Geometry check sheet. Reference: the model listing, model coordinates, mm. A direction names the side the tool comes from. Give positions to 0.01 mm unless a question says otherwise; leave off trailing zeros. Loops run counter-clockwise (first coordinate to the right, second up) from the corner with the lowest first, then second, coordinate; pieces in that order, holes last.
1. Cross-section at B-B, the plane x = 11.2. Record the cut outline in (y, z).
2. Material ranges on L1, parallel to Y at x = 8.5, z = 2; L2, parallel to Z at x = -11.2, y = 2.35 (3 decimals); L3, parallel to X at y = 2.35, z = 0, recorded low to high.
3. Go/stop test with flat-tipped pins: pin 1 Ø2.5 at (x, z) = (11.2, 0) entering from +Y; pin 2 Ø3 at (y, z) = (-9.5, -14) entering from -X; pin 3 Ø1 at (x, y) = (7.5, 2) entering from -Z; pin 4 Ø1.5 at (x, y) = (18, 2.5) entering from -Z. Record where each tip stops, or that it passes through.
4. Cross-section at C-C, the plane y = 1.5. State how many separate pieces and enclosed holes the cut face has, plus the area to 3 significant figures.
5. Tool access check on faces 5 (the flat face through (1, -9, -4)), 6 (the flat face through (15, 5, -2)). Record the directions out of +Z, -Z, +X, -X, +Y, -Y that give a thin tool (end or side, any length) a straight path to the whole face; none if there is none.
6. Cross-section at A-A, the plane x = -7.5. Record the cut outline in (y, z), plus the area to 3 significant figures.
7. Release check for a two-part mould opening along Z. For faces 1 (the cylindrical face through (9.614, 2.516, 0.208)), 2 (the cylindrical face through (-13.859, -8.516, 2.797)), 3 (the cylindrical face through (-13.859, 2.584, -2.797)), 4 (the cylindrical face through (-9.614, 2.516, -0.208)) record: +Z half, -Z half, draft (parallel to the pull), parting line (faces both ways), or undercut.
from build123d import *
from build123d.topology import SkipClean

# Parameters (mm, degrees)
SKETCH_1_W               = 30
SKETCH_1_H               = 8
SKETCH_1_R               = 1.6
EXTRUDE_1_DEPTH          = 5
EXTRUDE_2_DEPTH          = 5
EXTRUDE_START            = 11
SKETCH_3_R               = 1.6
EXTRUDE_3_DEPTH          = 11
CUT_EXTRUDE_1_DEPTH      = 0.1
CUT_EXTRUDE_1_DEPTH_BACK = 6.1
FILLET_1_R               = 4
FILLET_2_R               = 4
CUT_EXTRUDE_2_DEPTH      = 16
FILLET_3_R               = 3
FILLET_4_R               = 5


# Some blends are built 0.0001 mm under size
with BuildPart() as part:
    # 草图1 → 凸台-拉伸1 (new body)
    with BuildSketch(Plane(origin=(0, 0, 0), x_dir=(1, 0, 0), z_dir=(0, 1, 0))):
        Rectangle(SKETCH_1_W, SKETCH_1_H)
        with Locations(Location((-11.2, 0, 0), (0, 0, 270))):
            Circle(SKETCH_1_R, mode=Mode.SUBTRACT)
        with Locations(Location((11.2, 0, 0), (0, 0, 90))):
            Circle(SKETCH_1_R, mode=Mode.SUBTRACT)
    extrude(amount=EXTRUDE_1_DEPTH)

    # 草图2 → 凸台-拉伸2 (add)
    with BuildSketch(Plane(origin=(0, 5, 0), x_dir=(1, 0, 0), z_dir=(0, 1, 0))):
        Polygon((15, 4), (41.779934935, 17.521652446), (44.998681359, 11.146853201), (15, -4), align=None)
    extrude(amount=-EXTRUDE_2_DEPTH)

    # 草图3 → 凸台-拉伸3 (add)
    with SkipClean():  # the faces are left unmerged after this step: merging them gives an invalid solid
        with BuildSketch(Plane.XZ.offset(EXTRUDE_START)):
            Polygon((-15, -4), (15, -4), (41.779934935, -17.521652446), (44.998681359, -11.146853201), (15, 4), (-15, 4), align=None)
            with Locations(Location((-11.2, 0, 0), (0, 0, 270))):
                Circle(SKETCH_3_R, mode=Mode.SUBTRACT)
            with Locations(Location((11.2, 0, 0), (0, 0, 270))):
                Circle(SKETCH_3_R, mode=Mode.SUBTRACT)
        extrude(amount=-EXTRUDE_3_DEPTH)

    # 草图4 → 切除-拉伸1 (cut, two sides: drawn at the far end of the back side and taken through both)
    with BuildSketch(Plane(origin=(0, 0, 0), x_dir=(1, 0, 0), z_dir=(0, 1, 0)).offset(-CUT_EXTRUDE_1_DEPTH_BACK)):
        Polygon((17.677993493, 5.352165245), (20.899244527, -1.027594436), (19.919281017, -1.51616991), (15, -4), (-15, -4), (-15, 4), (15, 4), align=None)
    extrude(amount=CUT_EXTRUDE_1_DEPTH + CUT_EXTRUDE_1_DEPTH_BACK, mode=Mode.SUBTRACT)

    # 圆角1
    fillet_1_edges = [part.edges().sort_by_distance(p)[0] for p in [
        (-15, -8.55, -4),
        (-15, 2.55, -4),
        (-15, -8.55, 4),
        (-15, 2.55, 4),
    ]]
    fillet(fillet_1_edges, radius=FILLET_1_R - 0.0001)  # a hair under: the kernel refuses the full size

    # 圆角2
    # the kernel refuses this fillet: 4 mm, written as the material it takes off along each edge
    with BuildSketch(Plane(origin=(41.779934935, 15, -17.521652446), x_dir=(-0.8926644978329522, 0, 0.45072174820907335), z_dir=(0, -1, 0)), Plane(origin=(44.998681359, -21, -11.146853201), x_dir=(-0.8926644978329524, 0, 0.450721748209073), z_dir=(0, 1, 0))) as fillet_2_piece_1:
        with BuildLine():
            CenterArc((FILLET_2_R, -FILLET_2_R), FILLET_2_R, 90, 90)
            Line((0, -FILLET_2_R), (0, 0))
            Line((0, 0), (FILLET_2_R, 0))
        make_face()
    extrude(amount=36, mode=Mode.SUBTRACT)

    # 草图5 → 切除-拉伸2 (cut)
    with BuildSketch(Plane(origin=(0, 5, 0), x_dir=(1, 0, 0), z_dir=(0, 1, 0))):
        with BuildLine():
            Line((20.896739918, -1.022634001), (41.428023368, 9.343966208))
            add(Edge.make_bspline(
                [(20.896739918, -1.022634001), (25.980191779, 4.72849772), (33.095529518, 10.551057562), (41.428023368, 9.343966208)],
                knots=[0, 0, 0, 0, 1, 1, 1, 1], degree=3))
        make_face()
    extrude(amount=-CUT_EXTRUDE_2_DEPTH, mode=Mode.SUBTRACT)

    # 圆角3
    fillet_3_edges = [part.edges().sort_by_distance(p)[0] for p in [
        (41.428023368, -3, -9.343966208),
    ]]
    fillet(fillet_3_edges, radius=FILLET_3_R)

    # 圆角4
    fillet_4_edges = [part.edges().sort_by_distance(p)[0] for p in [
        (15, -8.55, 4),
        (15, -8.55, -4),
        (15, 2.55, 4),
        (15, 2.55, -4),
    ]]
    fillet(fillet_4_edges, radius=FILLET_4_R)


solid = part.part
Result:
1. outline: (-11, -4) - (-6.1, -4) - (-6.1, -1.6) - (-11, -1.6) - close; (-11, 1.6) - (-6.1, 1.6) - (-6.1, 4) - (-11, 4) - close; (0.1, -4) - (5, -4) - (5, -1.6) - (0.1, -1.6) - close; (0.1, 1.6) - (5, 1.6) - (5, 4) - (0.1, 4) - close
2. L1: y = -11 to -6.1, 0.1 to 5
2. L2: z = -3.995 to -1.6, 1.6 to 3.995
2. L3: x = -15 to -12.8, -9.6 to 9.6, 12.8 to 21.82
3. pin 1: passes through
3. pin 2: stops at x = 31.83
3. pin 3: stops at z = -4
3. pin 4: stops at z = -5.89
4. separate pieces: 1
4. enclosed holes: 2
4. area: 392 mm2
5. face 5: -Z, -X, +Y, -Y
5. face 6: +Z, -Z, +X, -X, +Y
6. outline: (-11, -4) - (-6.1, -4) - (-6.1, 4) - (-11, 4) - close; (0.1, -4) - (5, -4) - (5, 4) - (0.1, 4) - close
6. area: 78.4 mm2
7. face 1: undercut
7. face 2: +Z half
7. face 3: -Z half
7. face 4: undercut
